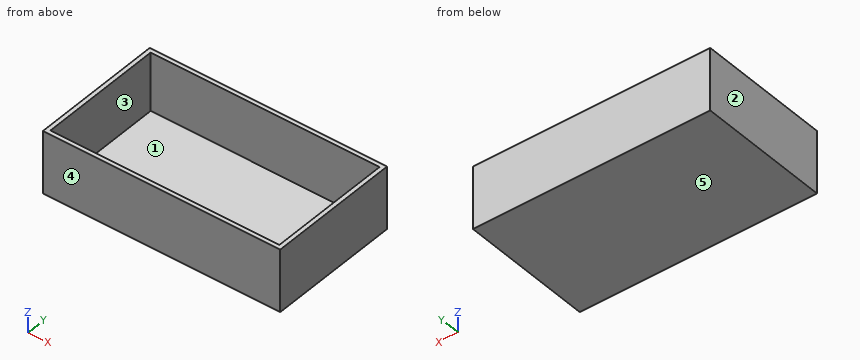
Solid Edge part; units mm, degrees
sketch "Sketch1" plane through (0, 0, 0) normal (0, 0, 1) x (1, 0, 0)
  line L0 (-55.2164, -24.0658) -> (54.7836, -24.0658)
  line L1 (54.7836, -24.0658) -> (54.7836, 35.9342)
  line L2 (54.7836, 35.9342) -> (-55.2164, 35.9342)
  line L3 (-55.2164, 35.9342) -> (-55.2164, -24.0658)
extrude "Protrusion1" add sketch "Sketch1" along normal blind 30
sketch "Sketch2" plane through (0, 0, 0) normal (0, 0, 1) x (1, 0, 0)
  line L0 (56.7836, -26.0658) -> (56.7836, 37.9342)
  line L1 (56.7836, 37.9342) -> (-57.2164, 37.9342)
  line L2 (-57.2164, 37.9342) -> (-57.2164, -26.0658)
  line L3 (-57.2164, -26.0658) -> (54.7836, -26.0658)
  line L4 (54.7836, -26.0658) -> (56.7836, -26.0658)
extrude "ExtrudedProtrusion_2" add sketch "Sketch2" along normal blind 30
sketch "Sketch3" plane through (-0.2164, 5.9342, 30) normal (0, 0, 1) x (1, 0, 0)
  line L0 (-55, 30) -> (55, 30)
  line L1 (55, 30) -> (55, -30)
  line L2 (55, -30) -> (-55, -30)
  line L3 (-55, -30) -> (-55, 30)
extrude "ExtrudedCutout_1" cut sketch "Sketch3" against normal blind 28
Read the model definition and answer for the solid it produces. Units are mm, in the model's axes. Face numbers are marked on the shaded views. A direction names the side the tool comes from. Give positions to 0.01 mm unless a question says otherwise; leave off trailing zeros. Order: outer loops, then holes, each group sorted by start corner. A loop starts at its lowest first (then second) coordinate and runs counter-clockwise, first axis right, second up.
(1) For the marked faces 1 and 2, determine the directions among +Z, -Z, +X, -X, +Y, -Y from which every point of the face is accessible in a straight line to the end or side of a thin tool.
(2) Straight lines are drawn through the part: L1, parallel to Y at x = -8.5, z = 27; L2, parallel to X at y = 10, z = 28.75; L3, parallel to Z at x = 16, y = 27. For each, find the intervals that lie inside material, in ascending order.
(3) Find section A-A (x = -0.5). Give the vertices of the cut face in (y, z).
(4) For a pull along Y with two mould halves and no side action, classify the marked faces 3, 4 and 5 as released by +Y, released by -Y, zero draft, split by the parting line, or undercut.
(5) Find section B-B (z = 21.5). Give the vertices of the cut face in (x, y).
(6) Find section C-C (y = 3.5). Give the vertices of the cut face in (x, z).
(7) Given pin 1 (10 mm diameter, centred on x = -4.5, y = 25, fed in from +Z), flat-ended and moving along its own axis, determine where the tip first touches the part or whether it passes through.
Result sheet:
1. face 1: +Z
1. face 2: +Z, -Z, -X, +Y, -Y
2. L1: y = -26.07 to -24.07, 35.93 to 37.93
2. L2: x = -57.22 to -55.22, 54.78 to 56.78
2. L3: z = 0 to 2
3. outline: (-26.07, 0) - (37.93, 0) - (37.93, 30) - (35.93, 30) - (35.93, 2) - (-24.07, 2) - (-24.07, 30) - (-26.07, 30) - close
4. face 3: undercut
4. face 4: released by -Y
4. face 5: zero draft
5. outline: (-57.22, -26.07) - (56.78, -26.07) - (56.78, 37.93) - (-57.22, 37.93) - close; hole (-55.22, -24.07) - (54.78, -24.07) - (54.78, 35.93) - (-55.22, 35.93) - close
6. outline: (-57.22, 0) - (56.78, 0) - (56.78, 30) - (54.78, 30) - (54.78, 2) - (-55.22, 2) - (-55.22, 30) - (-57.22, 30) - close
7. pin 1: stops at z = 2
